The model under review builds one solid part; all positions refer to its coordinate system, in mm. Face numbers are marked on the shaded views. A direction names the side the tool comes from. Coordinates: 2 decimals unless noted, no trailing zeros. Write each loop counter-clockwise with the first axis right and the second up, starting at its lowest first coordinate (ties: lowest second). Pieces come first, ordered by that corner, then holes. Notation, with made-up numbers: (12, -24) - (31, -24) arc R33 cw to (31, 10) - close; hole circle Ø2 at (68, 68). An arc over 180 degrees is marked (long way). Put each result on its own line as item: value.
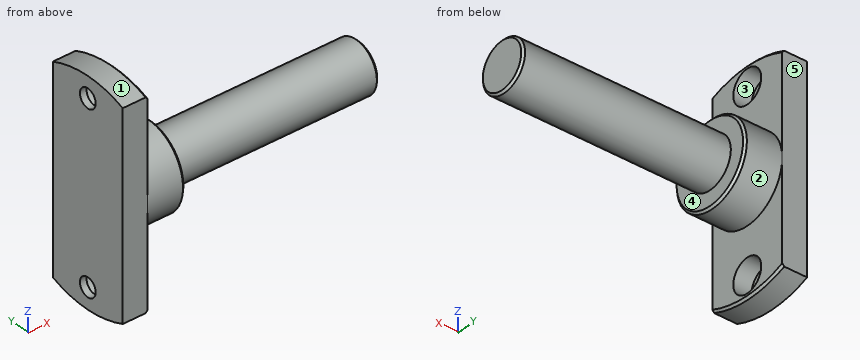
from build123d import *

# Parameters (mm, degrees)
CHANFREIN1_SIZE                                    = 0.5
CHAMBRAGE_POUR_VIS_T_TE_HEXAGONALE_M41_D           = 4.5
CHAMBRAGE_POUR_VIS_T_TE_HEXAGONALE_M41_CBORE_D     = 8
CHAMBRAGE_POUR_VIS_T_TE_HEXAGONALE_M41_CBORE_DEPTH = 4.4
ENL_V_MAT_EXTRU_2_DEPTH                            = 75.679314405
CHANFREIN3_SIZE                                    = 0.5


with BuildPart() as part:
    # Esquisse1 → Révolution1 (revolve)
    with BuildSketch(Plane.XY):
        Polygon((15, 6), (65, 6), (65, 0), (0, 0), (0, 26), (6, 26), (6, 10), (15, 10), align=None)
    revolve(axis=Axis((65, 0, 0), (-1, 0, 0)))

    # Chanfrein1
    chanfrein1_edges = [part.edges().sort_by_distance(p)[0] for p in [
        (6, -26, 0),
        (15, -10, 0),
    ]]
    chamfer(chanfrein1_edges, length=CHANFREIN1_SIZE)

    # Chambrage pour vis à tête hexagonale M41 (through all)
    with Locations(Plane(origin=(6, 0, 0), x_dir=(0, 0, -1), z_dir=(1, 0, 0))):
        with Locations((-21, 0), (21, 0)):
            CounterBoreHole(CHAMBRAGE_POUR_VIS_T_TE_HEXAGONALE_M41_D / 2, CHAMBRAGE_POUR_VIS_T_TE_HEXAGONALE_M41_CBORE_D / 2, CHAMBRAGE_POUR_VIS_T_TE_HEXAGONALE_M41_CBORE_DEPTH)

    # Esquisse11 → Enlèv. mat.-Extru.2 (cut, through all)
    with BuildSketch(Plane.ZY):
        with BuildLine():
            Line((24, -10), (-24, -10))
            ThreePointArc((-24, -10), (0, -26), (24, -10))
        make_face()
        with BuildLine():
            Line((24, 10), (-24, 10))
            ThreePointArc((-24, 10), (0, 26), (24, 10))
        make_face()
    extrude(amount=-ENL_V_MAT_EXTRU_2_DEPTH, mode=Mode.SUBTRACT)

    # Chanfrein3
    chanfrein3_edges = [part.edges().sort_by_distance(p)[0] for p in [
        (65, -6, 0),
    ]]
    chamfer(chanfrein3_edges, length=CHANFREIN3_SIZE)


solid = part.part
1. To check wall thickness, follow probe 1 along Y at (x, z) = (3, 21); probe 2 along Z at (x, y) = (11.5, 0.5); probe 3 along X at (y, z) = (4.5, 23.5). State the ranges of each line that lie inside material, in increasing order.
Determined:
probe 1: y = -10 to -4, 4 to 10
probe 2: z = -9.99 to 9.99
probe 3: x = 0 to 6
2. Consider section A-A on y = 0. Give the number of separate pieces and of enclosed holes in the cut face, plus the area to 3 significant figures.
Determined:
separate pieces: 3
enclosed holes: 0
area: 1,010 mm^2
3. The part is to be moulded in two halves that separate along Z. For the marked faces 1, 2 and 3, say which applies: +Z half, -Z half, draft (parallel to the pull), parting line (faces both ways), or undercut.
Determined:
face 1: +Z half
face 2: parting line
face 3: undercut
4. Consider section C-C on x = 48. State the section outline as (y, z) points.
Determined:
outline: circle Ø12 at (0, 0)
5. Consider section B-B on z = -21. State the section outline as (x, y) points, plus the area to 3 significant figures.
Determined:
outline: (0, -10) - (6, -10) - (6, -4) - (1.6, -4) - (1.6, -2.25) - (0, -2.25) - close; (0, 2.25) - (1.6, 2.25) - (1.6, 4) - (6, 4) - (6, 10) - (0, 10) - close
area: 77.6 mm^2
6. For pin 1 Ø6 at (x, y) = (31, 6) entering from -Z; pin 2 Ø9 at (y, z) = (1.5, -20) entering from +X; pin 3 Ø1.5 at (y, z) = (-5.5, 7) entering from +X, all flat-tipped, find the tip position at first contact; note any pin that passes through.
Determined:
pin 1: stops at z = -5.2
pin 2: stops at x = 6
pin 3: stops at x = 15
7. Machinability: for the marked faces 4 and 5, which of the approach directions +Z, -Z, +X, -X, +Y, -Y give a long, thin tool a straight path to every point of the face, cutting with its end or side? Answer none if there is none.
Determined:
face 4: +X
face 5: +Z, -Z, +X, -X, +Y
8. Consider section D-D on z = 20.5. State the section outline as (x, y) points, plus the area to 3 significant figures.
Determined:
outline: (0, -10) - (6, -10) - (6, -3.97) - (1.6, -3.97) - (1.6, -2.19) - (0, -2.19) - close; (0, 2.19) - (1.6, 2.19) - (1.6, 3.97) - (6, 3.97) - (6, 10) - (0, 10) - close
area: 78.1 mm^2
